Answer from the drawing. Dimensions are ordinates in mm from the lowest x, y and z of the part. A direction names the side the tool comes from. Round coordinates to 2 decimals unless told otherwise and drop trailing zeros. Order: outer loops, then holes, each group sorted by start corner. A loop starts at its lowest first (then second) coordinate and runs counter-clockwise, first axis right, second up.
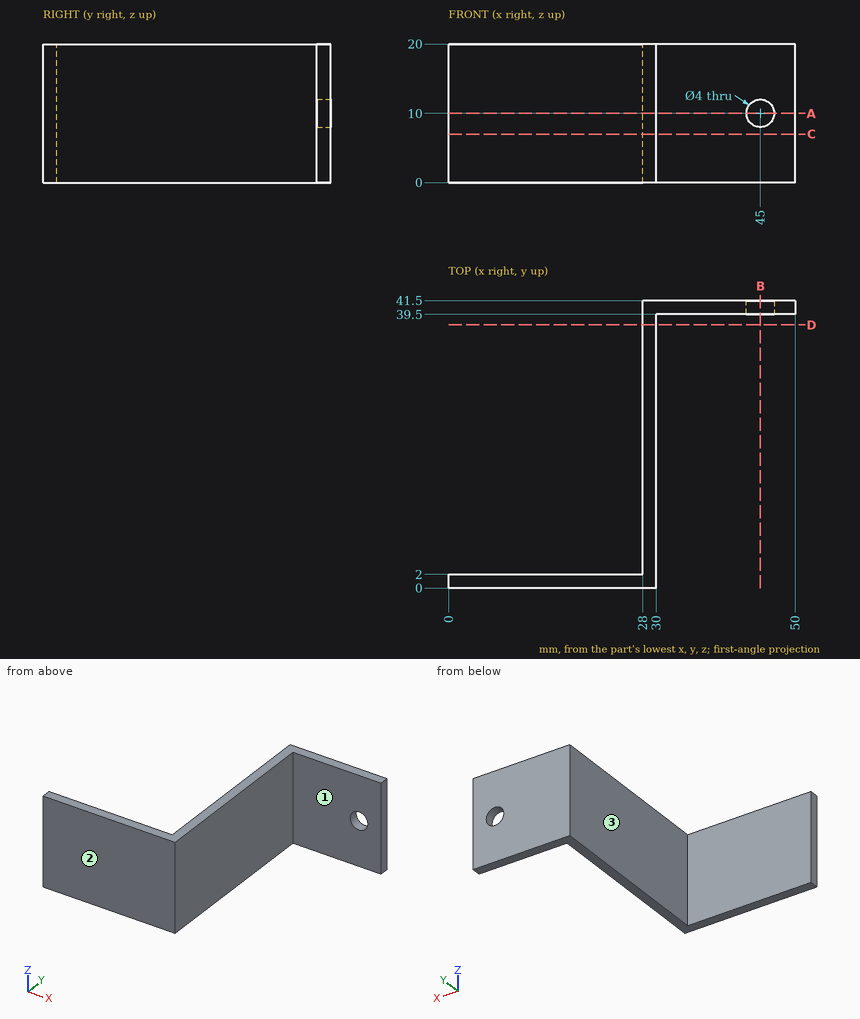
Q1. A cutting plane is placed at A-A, the plane z = 10. Give the vertices of the cut face in (x, y).
Outcome:
outline: (0, 0) - (30, 0) - (30, 39.5) - (43, 39.5) - (43, 41.5) - (28, 41.5) - (28, 2) - (0, 2) - close; (47, 39.5) - (50, 39.5) - (50, 41.5) - (47, 41.5) - close
Q2. Flat-ended cylindrical pins translate along their axes: pin 1 (10 mm diameter, centred on x = 12.5, z = 14.5, fed in from +Y); pin 2 (1.5 mm diameter, centred on y = 7.5, z = 6.5, fed in from -X); pin 3 (8 mm diameter, centred on y = 22.5, z = 4.5, fed in from +X). Find the tip coordinate at first contact, or state that the pin passes through.
Outcome:
pin 1: stops at y = 2
pin 2: stops at x = 28
pin 3: stops at x = 30
Q3. A cutting plane is placed at B-B, the plane x = 45. Give the vertices of the cut face in (y, z).
Outcome:
outline: (39.5, 0) - (41.5, 0) - (41.5, 8) - (39.5, 8) - close; (39.5, 12) - (41.5, 12) - (41.5, 20) - (39.5, 20) - close
Q4. For the marked faces 1, 2 and 3, determine the directions among +Z, -Z, +X, -X, +Y, -Y from which every point of the face is accessible in a straight line to the end or side of a thin tool.
Outcome:
face 1: +Z, -Z, +X, -Y
face 2: +Z, -Z, +X, -X, -Y
face 3: +Z, -Z, -X, +Y
Q5. A cutting plane is placed at C-C, the plane z = 7. Give the vertices of the cut face in (x, y).
Outcome:
outline: (0, 0) - (30, 0) - (30, 39.5) - (50, 39.5) - (50, 41.5) - (28, 41.5) - (28, 2) - (0, 2) - close
Q6. Straight lines are drawn through the part: probe 1 along X at (y, z) = (40.4, 10); probe 2 along Z at (x, y) = (45, 40); probe 3 along Y at (x, z) = (37.5, 2). For each, find the intervals that lie inside material, in ascending order.
Outcome:
probe 1: x = 28 to 43, 47 to 50
probe 2: z = 0 to 8, 12 to 20
probe 3: y = 39.5 to 41.5
Q7. A cutting plane is placed at D-D, the plane y = 38. Give the vertices of the cut face in (x, z), plus the area to 3 significant figures.
Outcome:
outline: (28, 0) - (30, 0) - (30, 20) - (28, 20) - close
area: 40.0 mm2
